Build history of the part. All positions in model axes, mm. A direction names the side the tool comes from. Give positions to 0.01 mm unless a question says otherwise; leave off trailing zeros. Write each loop counter-clockwise with the first axis right and the second up, starting at its lowest first coordinate (ties: lowest second). Pieces come first, ordered by that corner, then holes. Notation, with made-up numbers: (31.5, -3.75) -> (57.5, -3.75) arc R27 cw to (57.5, 30.25) -> close; hole circle Ø3 at (25.25, 30.25). An arc over 180 degrees is marked (long way). Put each result on its own line as item: value.
from build123d import *

# Parameters (mm, degrees)
SKETCH1_W           = 254
SKETCH1_H           = 254
SKETCH1_W_2         = 38.1
SKETCH1_H_2         = 38.1
BOSS_EXTRUDE1_DEPTH = 100
SKETCH2_W           = 252
SKETCH2_H           = 252
SKETCH2_W_2         = 40.1
SKETCH2_H_2         = 40.1
CUT_EXTRUDE1_DEPTH  = 98


with BuildPart() as part:
    # Sketch1 → Boss-Extrude1 (new body)
    with BuildSketch(Plane(origin=(0, 0, 0), x_dir=(1, 0, 0), z_dir=(0, 1, 0))):
        Rectangle(SKETCH1_W, SKETCH1_H)
        Rectangle(SKETCH1_W_2, SKETCH1_H_2, mode=Mode.SUBTRACT)
    extrude(amount=BOSS_EXTRUDE1_DEPTH)

    # Sketch2 → Cut-Extrude1 (cut)
    with BuildSketch(Plane(origin=(0, 99, 0), x_dir=(1, 0, 0), z_dir=(0, 1, 0))):
        Rectangle(SKETCH2_W, SKETCH2_H)
        Rectangle(SKETCH2_W_2, SKETCH2_H_2, mode=Mode.SUBTRACT)
    extrude(amount=-CUT_EXTRUDE1_DEPTH, mode=Mode.SUBTRACT)


solid = part.part
1) Wall check: L1, parallel to Z at x = -12, y = 4; L2, parallel to Z at x = 19.5, y = 77.5; L3, parallel to Y at x = 31, z = -12.5. Give the ranges that are in metal, low to high.
Filled sheet:
L1: -127 to -126, -20.05 to -19.05, 19.05 to 20.05, 126 to 127
L2: -127 to -126, -20.05 to 20.05, 126 to 127
L3: 0 to 1, 99 to 100
2) Pull direction Z, two halves, no side cores. Call faces 4 (the flat face through (-127, 49, 2)), 5 (the flat face through (-30, 99, -2)), 6 (the flat face through (-2, 49, 127)): released by +Z, released by -Z, zero draft, split by the parting line, or undercut.
Filled sheet:
face 4: zero draft
face 5: undercut
face 6: released by +Z
3) Slice it at C-C (x = -111). Write the cut outline in (y, z), plus the area to 3 significant figures.
Filled sheet:
outline: (0, -127) -> (100, -127) -> (100, 127) -> (0, 127) -> close; hole (1, -126) -> (99, -126) -> (99, 126) -> (1, 126) -> close
area: 704 mm2
4) Tool access for faces 1 (the flat face through (26, 100, -2)), 2 (the flat face through (19.05, 49, 0)), 3 (the flat face through (-126, 51, 2)): list every direction of +Z, -Z, +X, -X, +Y, -Y with a clear straight run to the whole face (end or side of a thin tool).
Filled sheet:
face 1: +Z, -Z, +X, -X, +Y
face 2: +Y, -Y
face 3: none
5) Slice it at A-A (x = 14.5). Write the cut outline in (y, z), plus the area to 3 significant figures.
Filled sheet:
outline: (0, -127) -> (100, -127) -> (100, -19.05) -> (0, -19.05) -> close; (0, 19.05) -> (100, 19.05) -> (100, 127) -> (0, 127) -> close; hole (1, -126) -> (99, -126) -> (99, -20.05) -> (1, -20.05) -> close; hole (1, 20.05) -> (99, 20.05) -> (99, 126) -> (1, 126) -> close
area: 824 mm2
6) Slice it at D-D (z = -85). Write the cut outline in (x, y).
Filled sheet:
outline: (-127, 0) -> (127, 0) -> (127, 100) -> (-127, 100) -> close; hole (-126, 1) -> (126, 1) -> (126, 99) -> (-126, 99) -> close
7) Slice it at B-B (z = -8.5). Write the cut outline in (x, y), plus the area to 3 significant figures.
Filled sheet:
outline: (-127, 0) -> (-19.05, 0) -> (-19.05, 100) -> (-127, 100) -> close; (19.05, 0) -> (127, 0) -> (127, 100) -> (19.05, 100) -> close; hole (-126, 1) -> (-20.05, 1) -> (-20.05, 99) -> (-126, 99) -> close; hole (20.05, 1) -> (126, 1) -> (126, 99) -> (20.05, 99) -> close
area: 824 mm2
